Here's how the part is built. I have some questions about the finished solid (model axes, mm). A direction names the side the tool comes from. Coordinates: 2 decimals unless noted, no trailing zeros. Order: outer loops, then holes, each group sorted by start corner. A loop starts at its lowest first (then second) coordinate and runs counter-clockwise, first axis right, second up. Notation, with made-up numbers: M 54,15 L 84,15 A20 ccw 84,43 Z; hole C 50,56 d7. An arc over 180 degrees is marked long. Answer as CSV lines item,"result". Start each with the question number.
```python
from build123d import *

# Parameters (mm, degrees)
EXTRUDE_2_DEPTH     = 15.2
SKETCH_4_W          = 12
SKETCH_4_H          = 10
EXTRUDE_3_DEPTH     = 9
SKETCH_5_R          = 2
EXTRUDE_4_DEPTH     = 1
SKETCH_6_R          = 1.5
EXTRUDE_5_DEPTH     = 9
CUT_EXTRUDE_START   = -8
CUT_EXTRUDE_2_DEPTH = 8
CHAMFER_1_SIZE      = 0.5
FILLET_1_R          = 1
SKETCH_8_R          = 3
EXTRUDE_6_DEPTH     = 3


with BuildPart() as part:
    # Эскиз3 → Бобышка-Вытянуть2 (new body)
    with BuildSketch(Plane(origin=(0, 0, 0), x_dir=(1, 0, 0), z_dir=(0, 1, 0))):
        with BuildLine():
            Line((-3.31662479, -5), (3.31662479, -5))
            ThreePointArc((3.31662479, -5), (6, 0), (3.31662479, 5))
            Line((3.31662479, 5), (-3.31662479, 5))
            ThreePointArc((-3.31662479, 5), (-6, 0), (-3.31662479, -5))
        make_face()
    extrude(amount=EXTRUDE_2_DEPTH)

    # Эскиз4 → Бобышка-Вытянуть3 (add)
    with BuildSketch(Plane(origin=(0, 15.2, 0), x_dir=(1, 0, 0), z_dir=(0, 1, 0))):
        Rectangle(SKETCH_4_W, SKETCH_4_H)
    extrude(amount=EXTRUDE_3_DEPTH)

    # Эскиз5 → Бобышка-Вытянуть4 (add)
    with BuildSketch(Plane(origin=(0, 24.2, 0), x_dir=(1, 0, 0), z_dir=(0, 1, 0))):
        with Locations(Location((0, 0, 0), (0, 0, 270))):
            Circle(SKETCH_5_R)
    extrude(amount=EXTRUDE_4_DEPTH)

    # Эскиз6 → Бобышка-Вытянуть5 (add)
    with BuildSketch(Plane(origin=(0, 25.2, 0), x_dir=(1, 0, 0), z_dir=(0, 1, 0))):
        with Locations(Location((0, 0, 0), (0, 0, 270))):
            Circle(SKETCH_6_R)
    extrude(amount=EXTRUDE_5_DEPTH)

    # Эскиз7 → Вырез-Вытянуть2 (cut)
    with BuildSketch(Plane(origin=(0, 34.2, 0), x_dir=(1, 0, 0), z_dir=(0, 1, 0)).offset(CUT_EXTRUDE_START)):
        with BuildLine():
            Line((-1.118033989, 1), (1.118033989, 1))
            ThreePointArc((1.118033989, 1), (0, 1.5), (-1.118033989, 1))
        make_face()
    extrude(amount=CUT_EXTRUDE_2_DEPTH, mode=Mode.SUBTRACT)

    # Фаска1
    chamfer_1_edges = [part.edges().sort_by_distance(p)[0] for p in [
        (-1.369306394, 34.2, 0.612372436),
        (0, 34.2, -1),
    ]]
    chamfer(chamfer_1_edges, length=CHAMFER_1_SIZE - 0.0001)  # a hair under: the kernel refuses the full size

    # Скругление1
    fillet_1_edges = [part.edges().sort_by_distance(p)[0] for p in [
        (-6, 24.2, 0),
        (0, 24.2, 5),
        (6, 24.2, 0),
        (0, 24.2, -5),
        (0, 0, -5),
        (6, 0, 0),
        (0, 0, 5),
        (-6, 0, 0),
    ]]
    fillet(fillet_1_edges, radius=FILLET_1_R - 0.0001)  # a hair under: the kernel refuses the full size

    # Эскиз8 → Бобышка-Вытянуть6 (add)
    with BuildSketch(Plane.XZ):
        with Locations(Location((0, 0, 0), (0, 0, 90))):
            Circle(SKETCH_8_R)
    extrude(amount=EXTRUDE_6_DEPTH)


solid = part.part
```
1) Will these pins go through, and if not, where does the flat tip stop? pin 1 Ø1.3 at (x, z) = (4.5, -2) entering from -Y; pin 2 Ø2.5 at (x, y) = (0, 31) entering from -Z; pin 3 Ø5 at (x, z) = (-3.5, 3) entering from +Y.
2) Suppose I cut it at C-C on y = 10.5. Please give me the cut outline in (x, z), plus the area to 3 significant figures.
3) Which directions (+Z, -Z, +X, -X, +Y, -Y) give clear straight access to the entire face, cutting with the end or side of a thin tool? Please do faces 1 (the face through (5, 15.2, -4)), 2 (the face through (-6, 8, 0)), 3 (the face through (5, 15.2, 4)), 4 (the face through (-0.9, -1.48, 2.86)).
4) I need wall thicknesses on line 1 (Z direction, x = -5, y = 1.5); line 2 (Y direction, x = -1.75, z = -2.25); line 3 (Y direction, x = 2.25, z = -4). Which ranges of each line are inside material? Lowest first, please. Write a range as [from, to].
5) Suppose I cut it at B-B on y = 27. Please give me the cut outline in (x, z).
6) Suppose I cut it at A-A on x = 0. Please give me the cut outline in (y, z).
Output:
1,pin 1,"y = 0"
1,pin 2,"z = -1"
1,pin 3,"y = 24.2"
2,outline,"M -3.32,-5 L 3.32,-5 A6 ccw 3.32,5 L -3.32,5 A6 ccw Z"
2,area,"104 mm²"
3,face 1,"-Z, +X, -Y"
3,face 2,"-X, -Y"
3,face 3,"+Z, +X, -Y"
3,face 4,"-Y"
4,line 1,"[-3.32, 3.32]"
4,line 2,"[-3, 24.2]"
4,line 3,"[0, 24.2]"
5,outline,"M -1.12,-1 L 1.12,-1 A1.5 ccw long Z"
6,outline,"M -3,-3 L 0,-3 L 0,-4 A1 ccw 1,-5 L 23.2,-5 A1 ccw 24.2,-4 L 24.2,-2 L 25.2,-2 L 25.2,-1.5 L 26.2,-1.5 L 26.2,-1 L 33.7,-1 L 34.2,-0.5 L 34.2,1 L 33.7,1.5 L 25.2,1.5 L 25.2,2 L 24.2,2 L 24.2,4 A1 ccw 23.2,5 L 1,5 A1 ccw 0,4 L 0,3 L -3,3 Z"
